```python
from build123d import *

# Parameters (mm, degrees)
SKETCH_R   = 4
SKETCH_R_2 = 3
SKETCH_R_3 = 4.05
PAD_DEPTH  = 4


with BuildPart() as part:
    # Sketch → Pad (new body)
    with BuildSketch(Plane.XZ):
        with BuildLine():
            ThreePointArc((-18.533333, -7.517683), (-4.421216, -19.505201), (13.480464, -14.774204))
            ThreePointArc((64.49, 5), (37.135878, -0.116509), (13.480464, -14.774204))
            Line((64.49, 5), (110.202041, 5))
            ThreePointArc((110.202041, 5), (120.002802, 1), (129.801962, 5.003923))
            ThreePointArc((129.801962, 5.003923), (133.464809, 6.395129), (135, 10))
            Line((135, 20), (135, 10))
            ThreePointArc((135, 20), (133.535534, 23.535534), (130, 25))
            Line((130, 25), (-19, 25))
            ThreePointArc((-37.518519, 28.555792), (-28.428404, 25.896994), (-19, 25))
            ThreePointArc((-37.518519, 28.555792), (-45.721006, 31.350796), (-54.165443, 33.296133))
            ThreePointArc((-54.165443, 33.296133), (-75.549225, 34.99014), (-97, 35))
            ThreePointArc((-97, 35), (-105.999524, 26.09252), (-97.185031, 17.001902))
            ThreePointArc((-52.210866, 12.81731), (-74.622366, 15.721932), (-97.185031, 17.001902))
            ThreePointArc((-29.649803, 4.989386), (-40.598863, 9.858688), (-52.210866, 12.81731))
            ThreePointArc((-18.533333, -7.517683), (-23.014081, -0.306462), (-29.649803, 4.989386))
        make_face()
        Circle(SKETCH_R, mode=Mode.SUBTRACT)
        with Locations((-97, 26)):
            Circle(SKETCH_R_2, mode=Mode.SUBTRACT)
        with Locations((120, 15)):
            Circle(SKETCH_R_3, mode=Mode.SUBTRACT)
    extrude(amount=PAD_DEPTH)


solid = part.part
```
Can you work these out from the model? Positions are in its coordinate system, mm. A direction names the side the tool comes from. Give positions to 0.01 mm unless a question says otherwise; leave off trailing zeros. Loops run counter-clockwise (first coordinate to the right, second up) from the corner with the lowest first, then second, coordinate; pieces in that order, holes last. Notation, with made-up numbers: M -8,4.5 L 36,4.5 A24 cw 36,29.5 Z; hole C 45.25,-1.5 d7. An arc over 180 degrees is marked long. Answer in a Markdown table with one row per item.
1. For pin 1 Ø1 at (x, z) = (-75, 15) entering from -Y; pin 2 Ø2 at (y, z) = (-3, 29) entering from -X, each with a flat end and sliding along its axis, tell me the tip position at first contact or that it passes through.
Taken from the geometry:
| item | result |
|---|---|
| pin 1 | passes through |
| pin 2 | stops at x = -105.77 |
2. Thinking about a two-plate mould opening in Z: for faces 4 (the cylindrical face through (-100, -2, 26)), 5 (the cylindrical face through (120, -2, 1)), 6 (the flat face through (13, 0, 14)), which applies, released by +Z, released by -Z, zero draft, split by the parting line, or undercut?
Taken from the geometry:
| item | result |
|---|---|
| face 4 | undercut |
| face 5 | released by -Z |
| face 6 | zero draft |
3. Suppose I cut it at A-A on x = 0. Write out the boundary of the cut face in (y, z), plus the area to 3 significant figures.
Taken from the geometry:
| item | result |
|---|---|
| outline | M -4,-20 L 0,-20 L 0,-4 L -4,-4 Z; M -4,4 L 0,4 L 0,25 L -4,25 Z |
| area | 148 mm² |
4. If I drill on line 1 along Z through (x, y) = (0, -1.8); line 2 along Z through (x, y) = (-97, -1.65); line 3 along Z through (x, y) = (90, -1.4), over which ranges is the centre line in solid material (lowest first)?
Taken from the geometry:
| item | result |
|---|---|
| line 1 | z = -20 to -4, 4 to 25 |
| line 2 | z = 17 to 23, 29 to 35 |
| line 3 | z = 5 to 25 |
5. Which directions (+Z, -Z, +X, -X, +Y, -Y) give clear straight access to the entire face, cutting with the end or side of a thin tool? Please do faces 1 (the flat face through (57, -2, 25)), 2 (the cylindrical face through (-75.25, -1.97, 34.98)), 3 (the cylindrical face through (37.502, -1.972, 0.024)).
Taken from the geometry:
| item | result |
|---|---|
| face 1 | +Z, +X, +Y, -Y |
| face 2 | +Z, +Y, -Y |
| face 3 | -Z, +Y, -Y |
6. Suppose I cut it at D-D on x = -88.5. Write out the boundary of the cut face in (y, z), plus the area to 3 significant figures.
Taken from the geometry:
| item | result |
|---|---|
| outline | M -4,16.7 L 0,16.7 L 0,35.2 L -4,35.2 Z |
| area | 74.0 mm² |
7. Suppose I cut it at B-B on x = 120. Write out the boundary of the cut face in (y, z).
Taken from the geometry:
| item | result |
|---|---|
| outline | M -4,1 L 0,1 L 0,10.95 L -4,10.95 Z; M -4,19.05 L 0,19.05 L 0,25 L -4,25 Z |
8. Suppose I cut it at C-C on z = 7.5. Write out the boundary of the cut face in (x, y).
Taken from the geometry:
| item | result |
|---|---|
| outline | M -34.67,-4 L 134.33,-4 L 134.33,0 L -34.67,0 Z |
